```python
from build123d import *

# Parameters (mm, degrees)
SKETCH_1_W                       = 36.5
SKETCH_1_H                       = 26
SM_BASE_FLANGE_1_DEPTH           = 2
SM_EDGE_FLANGE_1_STRIP_CUT_DEPTH = 26
SM_EDGE_FLANGE_1_DEPTH           = 26
SM_EDGE_FLANGE_2_STRIP_CUT_DEPTH = 26
SM_EDGE_FLANGE_2_DEPTH           = 26
SM_EDGE_FLANGE_3_STRIP_CUT_DEPTH = 26
SM_EDGE_FLANGE_3_DEPTH           = 26
SM_EDGE_FLANGE_4_STRIP_CUT_DEPTH = 26
SM_EDGE_FLANGE_4_DEPTH           = 26
CUT_EXTRUDE_1_DEPTH              = 2
CUT_EXTRUDE_START                = -2
CUT_EXTRUDE_2_DEPTH              = 2
SKETCH_28_R                      = 6
SKETCH_28_R_2                    = 1.5
CUT_EXTRUDE_3_DEPTH              = 2
SKETCH_33_R                      = 4
SKETCH_33_R_2                    = 1
SKETCH_33_R_3                    = 1.5
CUT_EXTRUDE_4_DEPTH              = 2
SKETCH_34_R                      = 1
SKETCH_34_R_2                    = 1.5
SKETCH_34_R_3                    = 4
CUT_EXTRUDE_5_DEPTH              = 2
SKETCH_35_R                      = 1.5
CUT_EXTRUDE_6_DEPTH              = 2
SKETCH_36_R                      = 1.5
CUT_EXTRUDE_7_DEPTH              = 2
SKETCH_37_R                      = 1.5
CUT_EXTRUDE_8_DEPTH              = 100


# Sheet-metal steps are written as plain solids
with BuildPart() as part:
    # Sketch 1 → 基体-法兰1 (new body)
    with BuildSketch(Plane.XY):
        with Locations((0.504940711, 5.522068511)):
            Rectangle(SKETCH_1_W, SKETCH_1_H)
    extrude(amount=-SM_BASE_FLANGE_1_DEPTH)

    # 边线-法兰1 strip (across the edge) → 边线-法兰1 strip cut (cut)
    with BuildSketch(Plane(origin=(18.754940711, -7.477931489, 0), x_dir=(-0.8660254037844364, 0, 0.5000000000000041), z_dir=(0, 1, 0))):
        Polygon((-8.835731855, 2.791911088), (-0.6317, -1.944688912), (0.3683, -0.212638104), (-7.835731855, 4.523961896), align=None)
    extrude(amount=SM_EDGE_FLANGE_1_STRIP_CUT_DEPTH, mode=Mode.SUBTRACT)

    # 边线-法兰1 section (across the edge) → 边线-法兰1 (add)
    with BuildSketch(Plane(origin=(18.754940711, -7.477931489, 0), x_dir=(-0.8660254037844364, 0, 0.5000000000000041), z_dir=(0, 1, 0))):
        with BuildLine():
            Line((-2, 0.425276208), (-2, 14.845299462))
            Line((-2, 14.845299462), (0, 14.845299462))
            Line((0, 14.845299462), (0, 0.425276208))
            ThreePointArc((0, 0.425276208), (0.098685688, 0.056976208), (0.3683, -0.212638104))
            Line((0.3683, -0.212638104), (-0.6317, -1.944688912))
            ThreePointArc((-0.6317, -1.944688912), (-1.63336512, -0.943023792), (-2, 0.425276208))
        make_face()
    extrude(amount=SM_EDGE_FLANGE_1_DEPTH)

    # 边线-法兰2 strip (across the edge) → 边线-法兰2 strip cut (cut)
    with BuildSketch(Plane(origin=(26.177590442, -7.477931489, 12.856406461), x_dir=(-1, 0, 0), z_dir=(0, 1, 0))):
        Polygon((-6.36996512, 7.03310323), (-1.63336512, -1.170928625), (0.098685688, -0.170928625), (-4.637914312, 8.03310323), align=None)
    extrude(amount=SM_EDGE_FLANGE_2_STRIP_CUT_DEPTH, mode=Mode.SUBTRACT)

    # 边线-法兰2 section (across the edge) → 边线-法兰2 (add)
    with BuildSketch(Plane(origin=(26.177590442, -7.477931489, 12.856406461), x_dir=(-1, 0, 0), z_dir=(0, 1, 0))):
        with BuildLine():
            Line((-2, 0.197371375), (-2, 44.464101615))
            Line((-2, 44.464101615), (0, 44.464101615))
            Line((0, 44.464101615), (0, 0.197371375))
            ThreePointArc((0, 0.197371375), (0.025099036, 0.006725267), (0.098685688, -0.170928625))
            Line((0.098685688, -0.170928625), (-1.63336512, -1.170928625))
            ThreePointArc((-1.63336512, -1.170928625), (-1.906752616, -0.510912824), (-2, 0.197371375))
        make_face()
    extrude(amount=SM_EDGE_FLANGE_2_DEPTH)

    # 边线-法兰3 strip (across the edge) → 边线-法兰3 strip cut (cut)
    with BuildSketch(Plane(origin=(-17.745059289, 18.522068511, 0), x_dir=(0.8660254037844365, 0, 0.500000000000004), z_dir=(0, -1, 0))):
        Polygon((-8.835731855, 2.791911088), (-0.6317, -1.944688912), (0.3683, -0.212638104), (-7.835731855, 4.523961896), align=None)
    extrude(amount=SM_EDGE_FLANGE_3_STRIP_CUT_DEPTH, mode=Mode.SUBTRACT)

    # 边线-法兰3 section (across the edge) → 边线-法兰3 (add)
    with BuildSketch(Plane(origin=(-17.745059289, 18.522068511, 0), x_dir=(0.8660254037844365, 0, 0.500000000000004), z_dir=(0, -1, 0))):
        with BuildLine():
            Line((-2, 0.425276208), (-2, 14.845299462))
            Line((-2, 14.845299462), (0, 14.845299462))
            Line((0, 14.845299462), (0, 0.425276208))
            ThreePointArc((0, 0.425276208), (0.098685688, 0.056976208), (0.3683, -0.212638104))
            Line((0.3683, -0.212638104), (-0.6317, -1.944688912))
            ThreePointArc((-0.6317, -1.944688912), (-1.63336512, -0.943023792), (-2, 0.425276208))
        make_face()
    extrude(amount=SM_EDGE_FLANGE_3_DEPTH)

    # 边线-法兰4 strip (across the edge) → 边线-法兰4 strip cut (cut)
    with BuildSketch(Plane(origin=(-25.167709019, 18.522068511, 12.856406461), x_dir=(1, 0, 0), z_dir=(0, -1, 0))):
        Polygon((-6.36996512, 7.03310323), (-1.63336512, -1.170928625), (0.098685688, -0.170928625), (-4.637914312, 8.03310323), align=None)
    extrude(amount=SM_EDGE_FLANGE_4_STRIP_CUT_DEPTH, mode=Mode.SUBTRACT)

    # 边线-法兰4 section (across the edge) → 边线-法兰4 (add)
    with BuildSketch(Plane(origin=(-25.167709019, 18.522068511, 12.856406461), x_dir=(1, 0, 0), z_dir=(0, -1, 0))):
        with BuildLine():
            Line((-2, 0.197371375), (-2, 44.464101615))
            Line((-2, 44.464101615), (0, 44.464101615))
            Line((0, 44.464101615), (0, 0.197371375))
            ThreePointArc((0, 0.197371375), (0.025099036, 0.006725267), (0.098685688, -0.170928625))
            Line((0.098685688, -0.170928625), (-1.63336512, -1.170928625))
            ThreePointArc((-1.63336512, -1.170928625), (-1.906752616, -0.510912824), (-2, 0.197371375))
        make_face()
    extrude(amount=SM_EDGE_FLANGE_4_DEPTH)

    # 草图20 → 切除-拉伸1 (cut)
    with BuildSketch(Plane.ZY.offset(-26.177590442)):
        with BuildLine():
            ThreePointArc((44.320508076, 18.522068511), (53.512896231, 14.714456667), (57.320508076, 5.522068511))
            Line((57.320508076, 5.522068511), (57.320508076, 18.522068511))
            Line((57.320508076, 18.522068511), (44.320508076, 18.522068511))
        make_face()
        with BuildLine():
            Line((57.320508076, -7.477931489), (57.320508076, 5.522068511))
            ThreePointArc((57.320508076, 5.522068511), (53.512896231, -3.670319644), (44.320508076, -7.477931489))
            Line((44.320508076, -7.477931489), (57.320508076, -7.477931489))
        make_face()
    extrude(amount=-CUT_EXTRUDE_1_DEPTH, mode=Mode.SUBTRACT)

    # 草图21 → 切除-拉伸2 (cut)
    with BuildSketch(Plane(origin=(-25.167709019, 0, 0), x_dir=(0, 0, -1), z_dir=(1, 0, 0)).offset(CUT_EXTRUDE_START)):
        with BuildLine():
            Line((-57.320508076, -7.477931489), (-44.320508076, -7.477931489))
            ThreePointArc((-44.320508076, -7.477931489), (-53.512896231, -3.670319644), (-57.320508076, 5.522068511))
            Line((-57.320508076, 5.522068511), (-57.320508076, -7.477931489))
        make_face()
        with BuildLine():
            ThreePointArc((-57.320508076, 5.522068511), (-53.512896231, 14.714456667), (-44.320508076, 18.522068511))
            Line((-44.320508076, 18.522068511), (-57.320508076, 18.522068511))
            Line((-57.320508076, 18.522068511), (-57.320508076, 5.522068511))
        make_face()
    extrude(amount=CUT_EXTRUDE_2_DEPTH, mode=Mode.SUBTRACT)

    # 草图28 → 切除-拉伸3 (cut)
    with BuildSketch(Plane.XY):
        with Locations((0.077660184, 5.906325961)):
            Circle(SKETCH_28_R)
        with Locations((7.148727996, 12.977393772)):
            Circle(SKETCH_28_R_2)
        with Locations((-6.993407628, -1.164741851)):
            Circle(SKETCH_28_R_2)
        with Locations((-6.993407628, 12.977393772)):
            Circle(SKETCH_28_R_2)
        with Locations((7.148727996, -1.164741851)):
            Circle(SKETCH_28_R_2)
    extrude(amount=-CUT_EXTRUDE_3_DEPTH, mode=Mode.SUBTRACT)

    # 草图33 → 切除-拉伸4 (cut)
    with BuildSketch(Plane(origin=(28.177590442, 0, 0), x_dir=(0, 0, -1), z_dir=(1, 0, 0))):
        with Locations((-44.320508076, 5.522068511)):
            Circle(SKETCH_33_R)
        with Locations((-39.370760607, 10.47181598)):
            Circle(SKETCH_33_R_2)
        with Locations((-39.370760607, 0.572321043)):
            Circle(SKETCH_33_R_2)
        with Locations((-49.270255544, 0.572321043)):
            Circle(SKETCH_33_R_2)
        with Locations((-49.270255544, 10.47181598)):
            Circle(SKETCH_33_R_2)
        with Locations((-44.320508076, 12.522068511)):
            Circle(SKETCH_33_R_3)
        with Locations((-37.320508076, 5.522068511)):
            Circle(SKETCH_33_R_3)
        with Locations((-44.320508076, -1.477931489)):
            Circle(SKETCH_33_R_3)
        with Locations((-51.320508076, 5.522068511)):
            Circle(SKETCH_33_R_3)
    extrude(amount=-CUT_EXTRUDE_4_DEPTH, mode=Mode.SUBTRACT)

    # 草图34 → 切除-拉伸5 (cut)
    with BuildSketch(Plane.ZY.offset(27.167709019).offset(CUT_EXTRUDE_START)):
        with Locations(Location((49.270255544, 10.47181598, 0), (0, 0, 180))):
            Circle(SKETCH_34_R)
        with Locations(Location((51.320508076, 5.522068511, 0), (0, 0, 180))):
            Circle(SKETCH_34_R_2)
        with Locations(Location((49.270255544, 0.572321043, 0), (0, 0, 180))):
            Circle(SKETCH_34_R)
        with Locations(Location((44.320508076, -1.477931489, 0), (0, 0, 180))):
            Circle(SKETCH_34_R_2)
        with Locations(Location((39.370760607, 0.572321043, 0), (0, 0, 180))):
            Circle(SKETCH_34_R)
        with Locations(Location((37.320508076, 5.522068511, 0), (0, 0, 180))):
            Circle(SKETCH_34_R_2)
        with Locations(Location((39.370760607, 10.47181598, 0), (0, 0, 180))):
            Circle(SKETCH_34_R)
        with Locations(Location((44.320508076, 12.522068511, 0), (0, 0, 180))):
            Circle(SKETCH_34_R_2)
        with Locations(Location((44.320508076, 5.522068511, 0), (0, 0, 180))):
            Circle(SKETCH_34_R_3)
    extrude(amount=CUT_EXTRUDE_5_DEPTH, mode=Mode.SUBTRACT)

    # 草图35 → 切除-拉伸6 (cut)
    with BuildSketch(Plane(origin=(15.798256341, 0, -9.121127551), x_dir=(-0.5000000000000041, 0, -0.8660254037844364), z_dir=(0.8660254037844363, 0, -0.500000000000004))):
        with Locations((-16.914072503, -1.477931489)):
            Circle(SKETCH_35_R)
        with Locations((-16.914072503, 12.522068511)):
            Circle(SKETCH_35_R)
    extrude(amount=-CUT_EXTRUDE_6_DEPTH, mode=Mode.SUBTRACT)

    # 草图36 → 切除-拉伸7 (cut)
    with BuildSketch(Plane(origin=(-15.040845274, 0, -8.683836068), x_dir=(-0.5000000000000041, 0, 0.8660254037844364), z_dir=(-0.8660254037844363, 0, -0.500000000000004))):
        with Locations((16.409131792, 12.522068511)):
            Circle(SKETCH_36_R)
        with Locations((16.409131792, -1.477931489)):
            Circle(SKETCH_36_R)
    extrude(amount=-CUT_EXTRUDE_7_DEPTH, mode=Mode.SUBTRACT)

    # 草图37 → 切除-拉伸8 (cut)
    with BuildSketch(Plane(origin=(28.177590442, 0, 0), x_dir=(0, 0, -1), z_dir=(1, 0, 0))):
        with Locations((-23.053777836, 5.522068511)):
            Circle(SKETCH_37_R)
    extrude(amount=-CUT_EXTRUDE_8_DEPTH, mode=Mode.SUBTRACT)


solid = part.part
```
Model file for the job. Use its own axes, mm. A direction names the side the tool comes from. Give positions to 0.01 mm unless a question says otherwise; leave off trailing zeros. Write each loop counter-clockwise with the first axis right and the second up, starting at its lowest first coordinate (ties: lowest second). Pieces come first, ordered by that corner, then holes. Notation, with made-up numbers: M 41,13.5 L 54,13.5 A15 ccw 54,31.5 Z; hole C 51.25,13 d5. An arc over 180 degrees is marked long. Use a Markdown table: item, result.
1) Drill centre lines: line 1 (X direction, y = -4.25, z = 35); line 2 (Z direction, x = 11, y = 7); line 3 (X direction, y = 10.25, z = 8). Where is each one in solid material? Low to high. Write a range as from..to.
Responses:
| item | result |
|---|---|
| line 1 | x = -27.17..-25.17, 26.18..28.18 |
| line 2 | z = -2..0 |
| line 3 | x = -24.67..-22.36, 23.37..25.68 |
2) Tool access for faces 3 (the cylindrical face through (27.2, -1, 42.9)), 4 (the flat face through (22.57, 5.34, 6.61)): list every direction of +Z, -Z, +X, -X, +Y, -Y with a clear straight run to the whole face (end or side of a thin tool).
Responses:
| item | result |
|---|---|
| face 3 | +X, -X |
| face 4 | +Z, +Y, -Y |
3) Cut at B-B (x = 4.5). List the corners of the cut face in (y, z), and give its area (3 significant figures).
Responses:
| item | result |
|---|---|
| outline | M -7.48,-2 L 1.85,-2 L 1.85,0 L -7.48,0 Z; M 9.96,-2 L 18.52,-2 L 18.52,0 L 9.96,0 Z |
| area | 35.8 mm2 |
4) Cut at A-A (z = 16). List the corners of the cut face in (x, y), and give its area (3 significant figures).
Responses:
| item | result |
|---|---|
| outline | M -27.17,-7.48 L -25.17,-7.48 L -25.17,18.52 L -27.17,18.52 Z; M 26.18,-7.48 L 28.18,-7.48 L 28.18,18.52 L 26.18,18.52 Z |
| area | 104 mm2 |
5) Cut at C-C (y = 3.25). Give the number of separate pieces and of enclosed holes in the cut face, and give its area (3 significant figures).
Responses:
| item | result |
|---|---|
| separate pieces | 4 |
| enclosed holes | 0 |
| area | 268 mm2 |
6) Pin check, flat tips, straight feed: pin 1 (2 mm diameter, centred on y = 0.5, z = 6, fed in from -X); pin 2 (5 mm diameter, centred on x = -8.5, y = 1, fed in from +Z). Stop position of each tip, or through.
Responses:
| item | result |
|---|---|
| pin 1 | stops at x = -24.1 |
| pin 2 | stops at z = 0 |
7) Cut at D-D (z = 47.5). List the corners of the cut face in (x, y), and give its area (3 significant figures).
Responses:
| item | result |
|---|---|
| outline | M -27.17,-7.08 L -25.17,-7.08 L -25.17,3.09 L -27.17,3.09 Z; M -27.17,7.95 L -25.17,7.95 L -25.17,18.13 L -27.17,18.13 Z; M 26.18,-7.08 L 28.18,-7.08 L 28.18,3.09 L 26.18,3.09 Z; M 26.18,7.95 L 28.18,7.95 L 28.18,18.13 L 26.18,18.13 Z |
| area | 81.4 mm2 |
8) Pull direction Y, two halves, no side cores. Call faces 1 (the flat face through (-21.56, 5.7, 6.61)), 2 (the cylindrical face through (-26.15, -1.93, 42.89)): +Y half, -Y half, draft (parallel to the pull), parting line (faces both ways), or undercut.
Responses:
| item | result |
|---|---|
| face 1 | draft |
| face 2 | undercut |
